Source: CAD feature listing. Evaluate the final solid. Frame: model axes, mm. A direction names the side the tool comes from. Round coordinates to 2 decimals unless told otherwise and drop trailing zeros. Write each loop counter-clockwise with the first axis right and the second up, starting at its lowest first coordinate (ties: lowest second). Pieces come first, ordered by that corner, then holes. Notation, with made-up numbers: (71.25, 56.5) -> (78.25, 56.5) arc R18 ccw to (78.25, 61.5) -> close; hole circle Ø10 at (-20.75, 62). An arc over 180 degrees is marked (long way). Return JSON: item names as keys, results as strings. Group by question number.
from build123d import *

# Parameters (mm, degrees)
SKETCH1_R           = 1.5
SKETCH1_W           = 5
SKETCH1_H           = 3
BOSS_EXTRUDE1_DEPTH = 2.8
FILLET1_R           = 5


with BuildPart() as part:
    # Sketch1 → Boss-Extrude1 (new body)
    with BuildSketch(Plane.XY):
        with BuildLine():
            Line((0.006174378, 4.000000753), (75.527864276, 4.000000258))
            ThreePointArc((75.527864276, 4.000000258), (80.000000039, 6), (84.472135776, 4.0000002))
            Line((84.472135776, 4.0000002), (115.000000079, 4))
            ThreePointArc((115.000000079, 4), (119, -5.2e-08), (114.999999974, -4))
            Line((114.999999974, -4), (84.472136134, -3.9999998))
            ThreePointArc((84.472136134, -3.9999998), (79.999999961, -6), (75.527863814, -3.999999742))
            Line((75.527863814, -3.999999742), (-0.007082675, -3.999999247))
            ThreePointArc((-0.007082675, -3.999999247), (-4.000000026, 0.006628527), (0.006174378, 4.000000753))
        make_face()
        with Locations((80, 0)):
            Circle(SKETCH1_R, mode=Mode.SUBTRACT)
        with Locations((115, 0)):
            Circle(SKETCH1_R, mode=Mode.SUBTRACT)
        Circle(SKETCH1_R, mode=Mode.SUBTRACT)
        with Locations((31.499999974, 0)):
            Rectangle(SKETCH1_W, SKETCH1_H, mode=Mode.SUBTRACT)
    extrude(amount=BOSS_EXTRUDE1_DEPTH)

    # Fillet1
    fillet1_edges = [part.edges().sort_by_distance(p)[0] for p in [
        (75.527864276, 4.000000258, 1.4),
        (84.472135776, 4.0000002, 1.4),
        (84.472136134, -3.9999998, 1.4),
        (75.527863814, -3.999999742, 1.4),
    ]]
    fillet(fillet1_edges, radius=FILLET1_R)


solid = part.part
Item 1: Cut plane C-C on y = 0. Output: boundary loops of the cut face in (x, z), and give its area (3 significant figures).
Item 2: Cut plane D-D on x = 98. Output: boundary loops of the cut face in (y, z).
Item 3: Pull-direction query (X, two-part tool) for faces 6 (the flat face through (34, 0, 1)), 7 (the flat face through (100, 4, 1)), 8 (the cylindrical face through (84.8, 4.24, 1.42)), 9 (the flat face through (31, -1.5, 1)); classes: +X half, -X half, draft (parallel to the pull), parting line (faces both ways), or undercut.
Item 4: First-contact query: pin 1 Ø0.8 at (x, z) = (30.5, 2) entering from +Y; pin 2 Ø1.4 at (x, z) = (31.5, 1) entering from -Y; pin 3 Ø1.8 at (x, y) = (80, 0) entering from -Z. Flat tips, straight axial feed; report the tip coordinate or a pass-through.
Item 5: Cut plane A-A on x = 80. Output: boundary loops of the cut face in (y, z).
Item 6: Cut plane B-B on z = 1.6. Output: boundary loops of the cut face in (x, y), and give its area (3 significant figures).
Item 7: Material intervals for probe 1 along Y at (x, z) = (0, 1.2); probe 2 along X at (y, z) = (-0.75, 2.15); probe 3 along Y at (x, z) = (113, 1.75), sorted ascending.
Item 8: Set-up query: faces 1 (the flat face through (29, 0, 1)), 2 (the cylindrical face through (119, 0, 1)), 3 (the flat face through (101, -4, 1)), 4 (the flat face through (37, -4, 1)), 5 (the flat face through (36, 4, 1)). Return all of +Z, -Z, +X, -X, +Y, -Y with unobstructed straight access to the full face (end or side cutting, diameter ignored); none if empty.
Here are the results:
{
 "1": {"outline": "(-4, 0) -> (-1.5, 0) -> (-1.5, 2.8) -> (-4, 2.8) -> close; (1.5, 0) -> (29, 0) -> (29, 2.8) -> (1.5, 2.8) -> close; (34, 0) -> (78.5, 0) -> (78.5, 2.8) -> (34, 2.8) -> close; (81.5, 0) -> (113.5, 0) -> (113.5, 2.8) -> (81.5, 2.8) -> close; (116.5, 0) -> (119, 0) -> (119, 2.8) -> (116.5, 2.8) -> close", "area": "305 mm^2"},
 "2": {"outline": "(-4, 0) -> (4, 0) -> (4, 2.8) -> (-4, 2.8) -> close"},
 "3": {"face 6": "undercut", "face 7": "draft", "face 8": "+X half", "face 9": "undercut"},
 "4": {"pin 1": "stops at y = 4", "pin 2": "stops at y = -4", "pin 3": "passes through"},
 "5": {"outline": "(-6, 0) -> (-1.5, 0) -> (-1.5, 2.8) -> (-6, 2.8) -> close; (1.5, 0) -> (6, 0) -> (6, 2.8) -> (1.5, 2.8) -> close"},
 "6": {"outline": "(-0.01, -4) -> (73.68, -4) arc R5 cw to (76.55, -4.91) arc R6 ccw to (83.45, -4.91) arc R5 cw to (86.32, -4) -> (115, -4) arc R4 ccw to (115, 4) -> (86.32, 4) arc R5 cw to (83.45, 4.91) arc R6 ccw to (76.55, 4.91) arc R5 cw to (73.68, 4) -> (0.01, 4) arc R4 ccw to start; hole circle Ø3 at (0, 0); hole (29, -1.5) -> (34, -1.5) -> (34, 1.5) -> (29, 1.5) -> close; hole circle Ø3 at (80, 0); hole circle Ø3 at (115, 0)", "area": "960 mm^2"},
 "7": {"probe 1": "y = -4 to -1.5, 1.5 to 4", "probe 2": "x = -3.93 to -1.3, 1.3 to 29, 34 to 78.7, 81.3 to 113.7, 116.3 to 118.93", "probe 3": "y = -4 to 4"},
 "8": {"face 1": "+Z, -Z", "face 2": "+Z, -Z, +X", "face 3": "+Z, -Z, +X, -Y", "face 4": "+Z, -Z, -X, -Y", "face 5": "+Z, -Z, -X, +Y"}
}
